Answer from the drawing. Dimensions are ordinates in mm from the lowest x, y and z of the part. A direction names the side the tool comes from. Give positions to 0.01 mm unless a question says otherwise; leave off trailing zeros. Order: outer loops, then holes, each group sorted by start corner. A loop starts at its lowest first (then second) coordinate and runs counter-clockwise, first axis right, second up. Notation, with made-up numbers: M -27,54.5 L 4,54.5 A9 cw 4,60.5 Z; hole C 40.25,56.25 d6. An arc over 180 degrees is marked long. One line per item, written item: value.
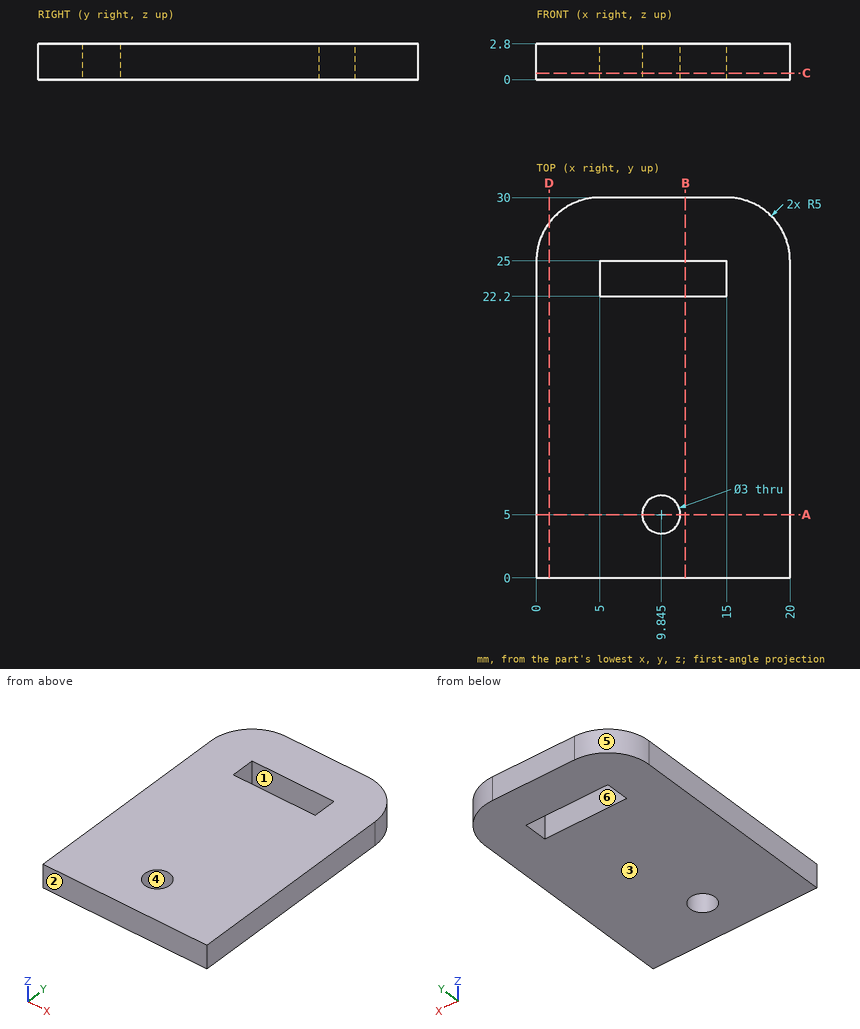
(1) Section D-D, the plane x = 1 is taken. Give the vertices of the cut face in (y, z), then the cut area to 3 significant figures.
Findings:
outline: M 0,0 L 28,0 L 28,2.8 L 0,2.8 Z
area: 78.4 mm^2
(2) Determine the mould class of the marked faces 3, 4, 5 and 6 for opening direction Y: pulls with the +Y half, pulls with the -Y half, needs draft (parallel to the pull), parting line crosses it, or undercut.
Findings:
face 3: needs draft
face 4: undercut
face 5: pulls with the +Y half
face 6: undercut
(3) Section C-C, the plane z = 0.5 is taken. Give the vertices of the cut face in (x, y) (1 decimal).
Findings:
outline: M 0,0 L 20,0 L 20,25 A5 ccw 15,30 L 5,30 A5 ccw 0,25 Z; hole M 5,22.2 L 15,22.2 L 15,25 L 5,25 Z; hole C 9.8,5 d3
(4) Section A-A, the plane y = 5 is taken. Give the vertices of the cut face in (x, z) (1 decimal).
Findings:
outline: M 0,0 L 8.3,0 L 8.3,2.8 L 0,2.8 Z; M 11.3,0 L 20,0 L 20,2.8 L 11.3,2.8 Z
(5) Which of the six approach directions +Z, -Z, +X, -X, +Y, -Y give full straight-line access (tool end or side, diameter ignored) to the marked faces 1 and 2?
Findings:
face 1: +Z, -Z
face 2: +Z, -Z, +X, -X, -Y
(6) Find the intervals of material crossed by probe 1 along Y at (x, z) = (13.25, 0.35); probe 2 along Y at (x, z) = (9, 1.4); probe 3 along X at (y, z) = (4.25, 0.6) (1 decimal), in increasing order. Write a range as from..to.
Findings:
probe 1: y = 0..22.2, 25..30
probe 2: y = 0..3.76, 6.24..22.2, 25..30
probe 3: x = 0..8.5, 11.1..20
(7) Section B-B, the plane x = 11.75 is taken. Give the vertices of the cut face in (y, z).
Findings:
outline: M 0,0 L 22.2,0 L 22.2,2.8 L 0,2.8 Z; M 25,0 L 30,0 L 30,2.8 L 25,2.8 Z
